```python
from build123d import *

# Parameters (mm, degrees)
BOSS_EXTRU_1_DEPTH           = 8
ESQUISSE14_R                 = 1.6
ENL_V_MAT_EXTRU_2_DEPTH      = 1
ENL_V_MAT_EXTRU_2_DEPTH_BACK = 9
ESQUISSE15_R                 = 3
ENL_V_MAT_EXTRU_3_DEPTH      = 4
ESQUISSE16_R                 = 2.5
BOSS_EXTRU_3_DEPTH           = 2
ESQUISSE17_R                 = 1.6
ENL_V_MAT_EXTRU_4_DEPTH      = 11


with BuildPart() as part:
    # Esquisse1 → Boss.-Extru.1 (new body)
    with BuildSketch(Plane.XY):
        with BuildLine():
            Line((2.96841177, 10.030192742), (146.96841177, 10.030192742))
            ThreePointArc((146.96841177, 10.030192742), (149.089732114, 10.908872398), (149.96841177, 13.030192742))
            Line((149.96841177, 13.030192742), (149.96841177, 97.09690847))
            ThreePointArc((149.96841177, 97.09690847), (149.301594422, 98.982712998), (147.597572626, 100.030192742))
            Line((147.597572626, 100.030192742), (2.96841177, 100.030192742))
            ThreePointArc((2.96841177, 100.030192742), (0.847091427, 99.151513085), (-0.03158823, 97.030192742))
            Line((-0.03158823, 97.030192742), (-0.03158823, 13.030192742))
            ThreePointArc((-0.03158823, 13.030192742), (0.847091427, 10.908872398), (2.96841177, 10.030192742))
        make_face()
    extrude(amount=BOSS_EXTRU_1_DEPTH)

    # Esquisse14 → Enlèv. mat.-Extru.2 (cut, two sides)
    with BuildSketch(Plane.XY.offset(8)) as enl_v_mat_extru_2_sk:
        with Locations((12.96841177, 97.530192742)):
            Circle(ESQUISSE14_R)
        with Locations((74.96841177, 97.530192742)):
            Circle(ESQUISSE14_R)
        with Locations((136.96841177, 97.530192742)):
            Circle(ESQUISSE14_R)
        with Locations((136.96841177, 55.030192742)):
            Circle(ESQUISSE14_R)
        with Locations((74.96841177, 55.030192742)):
            Circle(ESQUISSE14_R)
        with Locations((12.96841177, 55.030192742)):
            Circle(ESQUISSE14_R)
        with Locations((12.96841177, 12.530192742)):
            Circle(ESQUISSE14_R)
        with Locations((74.96841177, 12.530192742)):
            Circle(ESQUISSE14_R)
        with Locations((136.96841177, 12.530192742)):
            Circle(ESQUISSE14_R)
    extrude(amount=ENL_V_MAT_EXTRU_2_DEPTH, mode=Mode.SUBTRACT)
    extrude(enl_v_mat_extru_2_sk.sketch, amount=-ENL_V_MAT_EXTRU_2_DEPTH_BACK, mode=Mode.SUBTRACT)

    # Esquisse15 → Enlèv. mat.-Extru.3 (cut)
    with BuildSketch(Plane.XY.offset(8)):
        with Locations((12.96841177, 97.530192742)):
            Circle(ESQUISSE15_R)
        with Locations((12.96841177, 12.530192742)):
            Circle(ESQUISSE15_R)
        with Locations((74.96841177, 12.530192742)):
            Circle(ESQUISSE15_R)
        with Locations((136.96841177, 12.530192742)):
            Circle(ESQUISSE15_R)
        with Locations((136.96841177, 55.030192742)):
            Circle(ESQUISSE15_R)
        with Locations((74.96841177, 55.030192742)):
            Circle(ESQUISSE15_R)
        with Locations((12.96841177, 55.030192742)):
            Circle(ESQUISSE15_R)
        with Locations((74.96841177, 97.530192742)):
            Circle(ESQUISSE15_R)
        with Locations((136.96841177, 97.530192742)):
            Circle(ESQUISSE15_R)
    extrude(amount=-ENL_V_MAT_EXTRU_3_DEPTH, mode=Mode.SUBTRACT)

    # Esquisse16 → Boss.-Extru.3 (add)
    with BuildSketch(Plane(origin=(0, 0, 0), x_dir=(-1, 0, 0), z_dir=(0, 0, -1))):
        with Locations((-136.96841177, 97.530192742)):
            Circle(ESQUISSE16_R)
        with Locations((-74.96841177, 97.530192742)):
            Circle(ESQUISSE16_R)
        with Locations((-12.96841177, 97.530192742)):
            Circle(ESQUISSE16_R)
        with Locations((-12.96841177, 55.030192742)):
            Circle(ESQUISSE16_R)
        with Locations((-74.96841177, 55.030192742)):
            Circle(ESQUISSE16_R)
        with Locations((-136.96841177, 55.030192742)):
            Circle(ESQUISSE16_R)
        with Locations((-136.96841177, 12.530192742)):
            Circle(ESQUISSE16_R)
        with Locations((-74.96841177, 12.530192742)):
            Circle(ESQUISSE16_R)
        with Locations((-12.96841177, 12.530192742)):
            Circle(ESQUISSE16_R)
    extrude(amount=BOSS_EXTRU_3_DEPTH)

    # Esquisse17 → Enlèv. mat.-Extru.4 (cut, through all)
    with BuildSketch(Plane(origin=(0, 0, -2), x_dir=(-1, 0, 0), z_dir=(0, 0, -1))):
        with Locations((-136.96841177, 97.530192742)):
            Circle(ESQUISSE17_R)
        with Locations((-136.96841177, 55.030192742)):
            Circle(ESQUISSE17_R)
        with Locations((-136.96841177, 12.530192742)):
            Circle(ESQUISSE17_R)
        with Locations((-74.96841177, 12.530192742)):
            Circle(ESQUISSE17_R)
        with Locations((-74.96841177, 55.030192742)):
            Circle(ESQUISSE17_R)
        with Locations((-74.96841177, 97.530192742)):
            Circle(ESQUISSE17_R)
        with Locations((-12.96841177, 97.530192742)):
            Circle(ESQUISSE17_R)
        with Locations((-12.96841177, 55.030192742)):
            Circle(ESQUISSE17_R)
        with Locations((-12.96841177, 12.530192742)):
            Circle(ESQUISSE17_R)
    extrude(amount=-ENL_V_MAT_EXTRU_4_DEPTH, mode=Mode.SUBTRACT)


solid = part.part
```
Read the model definition and answer for the solid it produces. Units are mm, in the model's axes. A direction names the side the tool comes from. Give positions to 0.01 mm unless a question says otherwise; leave off trailing zeros. Order: outer loops, then holes, each group sorted by start corner. A loop starts at its lowest first (then second) coordinate and runs counter-clockwise, first axis right, second up. Notation, with made-up numbers: (12, -40) -> (21, -40) arc R24 cw to (21, -10) -> close; hole circle Ø9 at (51, 57). An arc over 180 degrees is marked (long way). One line per item, written item: value. Start each with the question number.
(1) For a pull along Y with two mould halves and no side action, classify faces 4 (the flat face through (73, 98, -2)), 5 (the cylindrical face through (149.32, 98.96, 3.94)), 6 (the cylindrical face through (72.584, 13.281, -0.986)) as released by +Y, released by -Y, zero draft, split by the parting line, or undercut.
(2) The part is cut by section A-A (z = 5.75). Determine the outline of the cut face in (x, y), and give its area (3 significant figures).
(3) The part is cut by section C-C (x = 51). Determine the outline of the cut face in (y, z).
(4) Flat-ended cylindrical pins translate along their axes: P1, Ø3, axis at x = 136.97, y = 55.03, coming from the -Z side; P2, Ø4, axis at x = 12.97, y = 97.53, coming from the +Z side; P3, Ø5, axis at x = 19, y = 85.5, coming from the -Z side. Find the tip coordinate at first contact, or state that the pin passes through.
(5) Straight lines are drawn through the part: L1, parallel to Y at x = 76, z = 2.75; L2, parallel to Z at x = 75, y = 78.5; L3, parallel to Y at x = 137.5, z = 7. For each, find the intervals that lie inside material, in ascending order.
(6) A tool of negligible diameter and unlimited length cuts with its end or side. For faces 1 (the cylindrical face through (13.51, 95.09, -0.99)), 2 (the cylindrical face through (12.578, 58.005, 6.028)), 3 (the flat face through (135, 98, -2)), from which of +Z, -Z, +X, -X, +Y, -Y can it reach the whole face along a straight path? Write none if from no direction.
(7) The part is cut by section B-B (y = 42.5). Determine the outline of the cut face in (x, z).
Taken from the geometry:
1. face 4: zero draft
1. face 5: released by +Y
1. face 6: undercut
2. outline: (-0.03, 13.03) arc R3 ccw to (2.97, 10.03) -> (11.31, 10.03) arc R3 cw (long way) to (14.63, 10.03) -> (73.31, 10.03) arc R3 cw (long way) to (76.63, 10.03) -> (135.31, 10.03) arc R3 cw (long way) to (138.63, 10.03) -> (146.97, 10.03) arc R3 ccw to (149.97, 13.03) -> (149.97, 97.1) arc R3 ccw to (147.6, 100.03) -> (138.63, 100.03) arc R3 cw (long way) to (135.31, 100.03) -> (76.63, 100.03) arc R3 cw (long way) to (73.31, 100.03) -> (14.63, 100.03) arc R3 cw (long way) to (11.31, 100.03) -> (2.97, 100.03) arc R3 ccw to (-0.03, 97.03) -> close; hole circle Ø6 at (12.97, 55.03); hole circle Ø6 at (74.97, 55.03); hole circle Ø6 at (136.97, 55.03)
2. area: 13,200 mm^2
3. outline: (10.03, 0) -> (100.03, 0) -> (100.03, 8) -> (10.03, 8) -> close
4. P1: through
4. P2: z = 4
4. P3: z = 0
5. L1: 10.03 to 11.31, 13.75 to 53.81, 56.25 to 96.31, 98.75 to 100.03
5. L2: 0 to 8
5. L3: 15.48 to 52.08, 57.98 to 94.58
6. face 1: -Z
6. face 2: +Z
6. face 3: -Z, +X, -X, +Y, -Y
7. outline: (-0.03, 0) -> (149.97, 0) -> (149.97, 8) -> (-0.03, 8) -> close
